```python
from build123d import *

# Parameters (mm, degrees)
SKIZZE11_R                = 2.15
QUADRATISCH_20X20_1_DEPTH = 264


with BuildPart() as part:
    # Skizze11 → Quadratisch 20X20(1) (new body)
    with BuildSketch(Plane(origin=(-132, 0, 0), x_dir=(0, 0, -1), z_dir=(1, 0, 0))):
        with BuildLine():
            Line((3.3, -10), (8, -10))
            ThreePointArc((8, -10), (9.414213562, -9.414213562), (10, -8))
            Line((10, -8), (10, -3.3))
            ThreePointArc((10, -3.3), (9.765685425, -2.734314575), (9.2, -2.5))
            Line((9.2, -2.5), (8.500000004, -2.5))
            ThreePointArc((8.500000004, -2.5), (8.28786797, -2.587867966), (8.200000004, -2.8))
            Line((8.200000004, -2.8), (8.200000004, -4.91758839))
            ThreePointArc((8.200000004, -4.91758839), (7.686138526, -5.686636439), (6.7789845, -5.506192284))
            Line((6.7789845, -5.506192284), (4.52867966, -3.255887444))
            ThreePointArc((4.52867966, -3.255887444), (3.878361407, -2.282617399), (3.650000005, -1.134567104))
            Line((3.650000005, -1.134567104), (3.650000005, 1.134567116))
            ThreePointArc((3.650000005, 1.134567116), (3.878361407, 2.282617413), (4.528679661, 3.25588746))
            Line((4.528679661, 3.25588746), (6.778984505, 5.506192304))
            ThreePointArc((6.778984505, 5.506192304), (7.686138528, 5.686636458), (8.200000004, 4.917588412))
            Line((8.200000004, 4.917588412), (8.200000004, 2.8))
            ThreePointArc((8.200000004, 2.8), (8.28786797, 2.587867966), (8.500000004, 2.5))
            Line((8.500000004, 2.5), (9.2, 2.5))
            ThreePointArc((9.2, 2.5), (9.765685425, 2.734314575), (10, 3.3))
            Line((10, 3.3), (10, 8))
            ThreePointArc((10, 8), (9.414213562, 9.414213562), (8, 10))
            Line((8, 10), (3.3, 10))
            ThreePointArc((3.3, 10), (2.734314575, 9.765685425), (2.5, 9.2))
            Line((2.5, 9.2), (2.5, 8.5))
            ThreePointArc((2.5, 8.5), (2.587867966, 8.287867966), (2.8, 8.2))
            Line((2.8, 8.2), (4.91758839, 8.2))
            ThreePointArc((4.91758839, 8.2), (5.686636437, 7.686138523), (5.506192283, 6.778984499))
            Line((5.506192283, 6.778984499), (3.255887448, 4.528679664))
            ThreePointArc((3.255887448, 4.528679664), (2.282617404, 3.878361412), (1.134567108, 3.650000009))
            Line((1.134567108, 3.650000009), (-1.134567106, 3.650000009))
            ThreePointArc((-1.134567106, 3.650000009), (-2.282617404, 3.878361412), (-3.25588745, 4.528679666))
            Line((-3.25588745, 4.528679666), (-5.50619229, 6.778984506))
            ThreePointArc((-5.50619229, 6.778984506), (-5.686636444, 7.686138526), (-4.9175884, 8.2))
            Line((-4.9175884, 8.2), (-2.8, 8.2))
            ThreePointArc((-2.8, 8.2), (-2.587867966, 8.287867966), (-2.5, 8.5))
            Line((-2.5, 8.5), (-2.5, 9.2))
            ThreePointArc((-2.5, 9.2), (-2.734314575, 9.765685425), (-3.3, 10))
            Line((-3.3, 10), (-8, 10))
            ThreePointArc((-8, 10), (-9.414213562, 9.414213562), (-10, 8))
            Line((-10, 8), (-10, 3.3))
            ThreePointArc((-10, 3.3), (-9.765685425, 2.734314575), (-9.2, 2.5))
            Line((-9.2, 2.5), (-8.5, 2.5))
            ThreePointArc((-8.5, 2.5), (-8.287867966, 2.587867966), (-8.2, 2.8))
            Line((-8.2, 2.8), (-8.2, 4.9175884))
            ThreePointArc((-8.2, 4.9175884), (-7.686138522, 5.686636449), (-6.778984496, 5.506192294))
            Line((-6.778984496, 5.506192294), (-4.528679665, 3.255887463))
            ThreePointArc((-4.528679665, 3.255887463), (-3.878361412, 2.282617418), (-3.65000001, 1.134567123))
            Line((-3.65000001, 1.134567123), (-3.65000001, -1.134567106))
            ThreePointArc((-3.65000001, -1.134567106), (-3.878361412, -2.282617404), (-4.528679666, -3.25588745))
            Line((-4.528679666, -3.25588745), (-6.778984506, -5.50619229))
            ThreePointArc((-6.778984506, -5.50619229), (-7.686138526, -5.686636444), (-8.2, -4.9175884))
            Line((-8.2, -4.9175884), (-8.2, -2.8))
            ThreePointArc((-8.2, -2.8), (-8.287867966, -2.587867966), (-8.5, -2.5))
            Line((-8.5, -2.5), (-9.2, -2.5))
            ThreePointArc((-9.2, -2.5), (-9.765685425, -2.734314575), (-10, -3.3))
            Line((-10, -3.3), (-10, -8))
            ThreePointArc((-10, -8), (-9.414213562, -9.414213562), (-8, -10))
            Line((-8, -10), (-3.3, -10))
            ThreePointArc((-3.3, -10), (-2.734314575, -9.765685425), (-2.5, -9.2))
            Line((-2.5, -9.2), (-2.5, -8.5))
            ThreePointArc((-2.5, -8.5), (-2.587867966, -8.287867966), (-2.8, -8.2))
            Line((-2.8, -8.2), (-4.9175884, -8.2))
            ThreePointArc((-4.9175884, -8.2), (-5.686636449, -7.686138522), (-5.506192294, -6.778984496))
            Line((-5.506192294, -6.778984496), (-3.255887454, -4.528679656))
            ThreePointArc((-3.255887454, -4.528679656), (-2.282617409, -3.878361403), (-1.134567114, -3.650000001))
            Line((-1.134567114, -3.650000001), (1.134567112, -3.650000001))
            ThreePointArc((1.134567112, -3.650000001), (2.282617409, -3.878361403), (3.255887456, -4.528679657))
            Line((3.255887456, -4.528679657), (5.5061923, -6.778984501))
            ThreePointArc((5.5061923, -6.778984501), (5.686636454, -7.686138524), (4.917588408, -8.2))
            Line((4.917588408, -8.2), (2.8, -8.2))
            ThreePointArc((2.8, -8.2), (2.587867966, -8.287867966), (2.5, -8.5))
            Line((2.5, -8.5), (2.5, -9.2))
            ThreePointArc((2.5, -9.2), (2.734314575, -9.765685425), (3.3, -10))
        make_face()
        Circle(SKIZZE11_R, mode=Mode.SUBTRACT)
    extrude(amount=QUADRATISCH_20X20_1_DEPTH)


solid = part.part
```
Input: part model. Units: mm. Frame: model coordinates. Coordinates: 2 decimals unless noted, no trailing zeros. Answer in a Markdown table with one row per item.
1. Draft query along Y for faces 1 (the cylindrical face through (-1.85, 0.09, 2.15)), 2 (the flat face through (-2, -10, -6)), 3 (the flat face through (-2, 10, 6)). Return one class per face: pulls with the +Y half, pulls with the -Y half, needs draft (parallel to the pull), parting line crosses it, or undercut.
Response:
| item | result |
|---|---|
| face 1 | undercut |
| face 2 | pulls with the -Y half |
| face 3 | pulls with the +Y half |
2. Material intervals for line 1 (Y direction, x = 23, z = 0); line 2 (Y direction, x = 67, z = 4.5); line 3 (Z direction, x = -120, y = 5.5), sorted ascending.
Response:
| item | result |
|---|---|
| line 1 | y = -3.65 to -2.15, 2.15 to 3.65 |
| line 2 | y = -10 to -8.2, -5.77 to -3.23, 3.23 to 5.77, 8.2 to 10 |
| line 3 | z = -10 to -7.96, -6.77 to -4.23, 4.23 to 6.77, 7.96 to 10 |
3. First-contact query: pin 1 (0.7 mm diameter, centred on x = 26.5, y = 0.5, fed in from -Z); pin 2 (1.5 mm diameter, centred on x = 95, y = -1.5, fed in from +Z); pin 3 (1 mm diameter, centred on x = -10.5, z = -1.5, fed in from +Y). Flat tips, straight axial feed; report the tip coordinate or a pass-through.
Response:
| item | result |
|---|---|
| pin 1 | stops at z = -3.65 |
| pin 2 | stops at z = 3.87 |
| pin 3 | stops at y = 3.78 |
